Can you work these out from the model? Positions are in its coordinate system, mm. Round coordinates to 2 decimals unless told otherwise and drop trailing zeros. Write each loop counter-clockwise with the first axis right and the second up, starting at its lowest first coordinate (ties: lowest second). Pieces come first, ordered by that corner, then holes. Notation, with made-up numbers: M 14.25,1.25 L 27.25,1.25 A37 cw 27.25,38.25 Z; hole C 78,-24.5 d9. An arc over 180 degrees is marked long. Answer in a Markdown table with one row per item. Add a question column.
(1) Suppose I cut it at A-A, the plane x = 0. Write out the boundary of the cut face in (y, z) (3 decimals), then the cut area to 3 significant figures.
(2) Suppose I cut it at C-C, the plane z = -12.5. Write out the boundary of the cut face in (x, y) (3 decimals).
(3) If I drill on probe 1 along Z at (x, y) = (0, -2.35); probe 2 along X at (y, z) = (-2.6, -20.5); probe 3 along X at (y, z) = (-1.7, 0.5), over which ranges is the centre line in solid material (lowest first)?
(4) Suppose I cut it at B-B, the plane x = 3.25. Write out the boundary of the cut face in (y, z) (3 decimals), then the cut area to 3 significant figures.
(5) If we mould it in two halves opening along X, with no side actions, what happens to faces 1 (the face through (-0.32, -1.61, 35.4)), 2 (the face through (-6.636, -1.565, 4.919)), 3 (the face through (6.8, -1.6, 4.1)), 4 (the face through (-1.65, -1.61, -22.05))? For each: released by +X, released by -X, zero draft, split by the parting line, or undercut.
(6) Suppose I cut it at D-D, the plane y = -1.05. Write out the boundary of the cut face in (x, z).
from build123d import *

# Parameters (mm, degrees)
F1_DEPTH = 3.175
F2_R     = 7.62
F3_DEPTH = 3.176
F5_DEPTH = 3.175
F6_R     = 1.4652480926
F7_DEPTH = 3.176


with BuildPart() as f1:
    # F0 (on Front) → F1 (new body)
    with BuildSketch(Plane.XZ):
        Polygon((12.7, -25.4), (0, 38.1), (-12.7, -25.4), align=None)
    extrude(amount=F1_DEPTH)

    # F2 (on face) → F3 (cut, through all)
    with BuildSketch(Plane.XZ.offset(3.175)):
        with Locations((0, -14.6123587166)):
            Circle(F2_R)
    extrude(amount=-F3_DEPTH, mode=Mode.SUBTRACT)

    # F4 (on face) → F5 (join, through all)
    with BuildSketch(Plane.XZ.offset(3.175)):
        with BuildLine():
            ThreePointArc((0.739965088, 34.4001745601), (2.0409692947, 35.3180329573), (2.54, 36.83))
            ThreePointArc((2.54, 36.83), (-1.5119670427, 38.8709692947), (-0.739965088, 34.4001745601))
            Line((-0.739965088, 34.4001745601), (0, 38.1))
            Line((0, 38.1), (0.739965088, 34.4001745601))
        make_face()
    extrude(amount=-F5_DEPTH)

    # F6 (on face) → F7 (cut, through all)
    with BuildSketch(Plane.XZ.offset(3.175)):
        with Locations((0, 36.83)):
            Circle(F6_R)
    extrude(amount=-F7_DEPTH, mode=Mode.SUBTRACT)


solid = f1.part
Calculated:
| question | item | result |
|---|---|---|
| 1 | outline | M -3.175,-25.4 L 0,-25.4 L 0,-22.232 L -3.175,-22.232 Z; M -3.175,-6.992 L 0,-6.992 L 0,35.365 L -3.175,35.365 Z; M -3.175,38.295 L 0,38.295 L 0,39.37 L -3.175,39.37 Z |
| 1 | area | 148 mm² |
| 2 | outline | M -10.12,-3.175 L -7.321,-3.175 L -7.321,0 L -10.12,0 Z; M 7.321,-3.175 L 10.12,-3.175 L 10.12,0 L 7.321,0 Z |
| 3 | probe 1 | -25.4 to -22.23, -6.99 to 35.36, 38.3 to 39.37 |
| 3 | probe 2 | -11.72 to -4.84, 4.84 to 11.72 |
| 3 | probe 3 | -7.52 to 7.52 |
| 4 | outline | M -3.175,-25.4 L 0,-25.4 L 0,-21.505 L -3.175,-21.505 Z; M -3.175,-7.72 L 0,-7.72 L 0,21.85 L -3.175,21.85 Z |
| 4 | area | 106 mm² |
| 5 | face 1 | undercut |
| 5 | face 2 | released by -X |
| 5 | face 3 | released by +X |
| 5 | face 4 | undercut |
| 6 | outline | M -12.7,-25.4 L 12.7,-25.4 L 0.74,34.4 A2.54 ccw long -0.74,34.4 Z; hole C 0,-14.61 d15.24; hole C 0,36.83 d2.93 |
